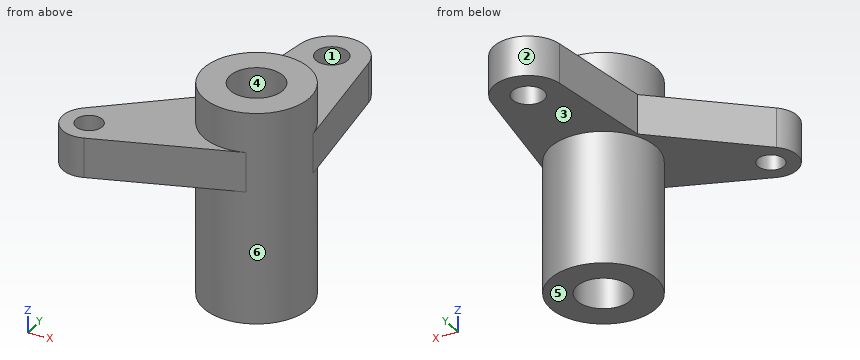
```python
from build123d import *

# Parameters (mm, degrees)
SKETCH_1_R      = 20
SKETCH_1_R_2    = 10
EXTRUDE_1_DEPTH = 80
EXTRUDE_START   = -15
SKETCH_1_3_R    = 13
SKETCH_1_3_R_2  = 6
SKETCH_1_3_R_3  = 10
SKETCH_1_3_R_4  = 5
EXTRUDE_2_DEPTH = 15


with BuildPart() as part:
    # Sketch 1 → Extrude 1 (new body)
    with BuildSketch(Plane.XY):
        Circle(SKETCH_1_R)
        Circle(SKETCH_1_R_2, mode=Mode.SUBTRACT)
    extrude(amount=-EXTRUDE_1_DEPTH)

    # Sketch 1_3 → Extrude 2 (add)
    # profile 1 of 5: a face of its own
    with BuildSketch(Plane.XY.offset(EXTRUDE_START)):
        with BuildLine():
            Line((-12.871969546, 51.82), (-18.742862332, 10.29804772))
            Line((-18.742862332, 10.29804772), (-12.982504947, 15.213630905))
            ThreePointArc((-12.982504947, 15.213630905), (7.081980571, 18.704158661), (19.803030071, 2.8))
            Line((19.803030071, 2.8), (12.871969546, 51.82))
            ThreePointArc((12.871969546, 51.82), (12.967952886, 50.912248842), (13, 50))
            ThreePointArc((13, 50), (-0.912248842, 37.032047114), (-12.871969546, 51.82))
        make_face()
    # profile 2 of 5: a face of its own
    with BuildSketch(Plane.XY.offset(EXTRUDE_START)):
        with BuildLine():
            Line((-12.982504947, 15.213630905), (-18.742862332, 10.29804772))
            Line((-18.742862332, 10.29804772), (-19.803030071, 2.8))
            ThreePointArc((-19.803030071, 2.8), (-17.528473541, 9.630815923), (-12.982504947, 15.213630905))
        make_face()
    # profile 3 of 5: a face of its own
    with BuildSketch(Plane.XY.offset(EXTRUDE_START)):
        with Locations((0, 50)):
            Circle(SKETCH_1_3_R)
        with Locations((0, 50)):
            Circle(SKETCH_1_3_R_2, mode=Mode.SUBTRACT)
    # profile 4 of 5: a face of its own
    with BuildSketch(Plane.XY.offset(EXTRUDE_START)):
        with BuildLine():
            Line((-18.742862332, 10.29804772), (-54.122649682, -19.893184548))
            ThreePointArc((-54.122649682, -19.893184548), (-43.442872691, -18.419456934), (-37.631397208, -27.5))
            ThreePointArc((-37.631397208, -27.5), (-39.463757039, -33.269718716), (-44.289328021, -36.924997271))
            Line((-44.289328021, -36.924997271), (6.684138374, -18.849994541))
            ThreePointArc((6.684138374, -18.849994541), (-12.657286271, -15.485254414), (-19.803030071, 2.8))
            Line((-19.803030071, 2.8), (-18.742862332, 10.29804772))
        make_face()
    # profile 5 of 5: a face of its own
    with BuildSketch(Plane.XY.offset(EXTRUDE_START)):
        with Locations((-47.631397208, -27.5)):
            Circle(SKETCH_1_3_R_3)
        with Locations((-47.631397208, -27.5)):
            Circle(SKETCH_1_3_R_4, mode=Mode.SUBTRACT)
    extrude(amount=-EXTRUDE_2_DEPTH)


solid = part.part
```
Could you check a few things on this model? Use its own coordinates, in mm. Face numbers are marked on the shaded views. A direction names the side the tool comes from. Coordinates: 2 decimals unless noted, no trailing zeros. Write each loop counter-clockwise with the first axis right and the second up, starting at its lowest first coordinate (ties: lowest second). Pieces come first, ordered by that corner, then holes. Notation, with made-up numbers: (50, 62.25) -> (101, 62.25) arc R37 ccw to (101, 101.25) -> close; hole circle Ø11 at (16, 32). An arc over 180 degrees is marked (long way). One line per question, with ' | ' between items. Start each with the question number.
1. If we section it at A-A (z = -25): Please give me the cut outline in (x, y) (3 decimals), and give its area (3 significant figures).
2. Thinking about a two-plate mould opening in Y: for the marked faces 1, 2, 3 and 4, which applies, pulls with the +Y half, pulls with the -Y half, needs draft (parallel to the pull), parting line crosses it, or undercut?
3. Please list where these lines run through material, in increasing order: line 1 along Y through (x, z) = (0, -42); line 2 along X through (y, z) = (-1, -42); line 3 along X through (y, z) = (47.5, -19).
4. Will these pins go through, and if not, where does the flat tip stop? P1, Ø10, axis at x = -20.5, y = 17, coming from the -Z side; P2, Ø4, axis at x = -8.5, z = -10.5, coming from the +Y side; P3, Ø12, axis at y = -13, z = -13, coming from the -X side.
5. For the marked faces 5 and 6, which set-ups out of +Z, -Z, +X, -X, +Y, -Y let a thin tool reach every point of the face, with its end or its side?
6. If we section it at B-B (y = 50): Please give me the cut outline in (x, z), and give its area (3 significant figures).
7. If we section it at D-D (x = 0): Please give me the cut outline in (y, z), and give its area (3 significant figures).
8. If we section it at C-C (z = -6): Please give me the cut outline in (x, y), and give its area (3 significant figures).
Return value:
1) outline: (-54.123, -19.893) arc R10 ccw to (-44.289, -36.925) -> (6.684, -18.85) arc R20 ccw to (19.803, 2.8) -> (12.872, 51.82) arc R13 ccw to (-12.872, 51.82) -> (-18.743, 10.298) -> close; hole circle Ø10 at (-47.631, -27.5); hole circle Ø20 at (0, 0); hole circle Ø12 at (0, 50) | area: 3,250 mm²
2) face 1: undercut | face 2: pulls with the +Y half | face 3: needs draft | face 4: undercut
3) line 1: y = -20 to -10, 10 to 20 | line 2: x = -19.97 to -9.95, 9.95 to 19.97 | line 3: x = -13.48 to -5.45, 5.45 to 13.48
4) P1: stops at z = -30 | P2: stops at y = 18.91 | P3: stops at x = -52.67
5) face 5: -Z, +X, -X, +Y, -Y | face 6: none
6) outline: (-13.13, -30) -> (-6, -30) -> (-6, -15) -> (-13.13, -15) -> close; (6, -30) -> (13.13, -30) -> (13.13, -15) -> (6, -15) -> close | area: 214 mm²
7) outline: (-21.22, -30) -> (-20, -30) -> (-20, -80) -> (-10, -80) -> (-10, 0) -> (-20, 0) -> (-20, -15) -> (-21.22, -15) -> close; (10, -80) -> (20, -80) -> (20, -30) -> (44, -30) -> (44, -15) -> (20, -15) -> (20, 0) -> (10, 0) -> close; (56, -30) -> (63, -30) -> (63, -15) -> (56, -15) -> close | area: 2,080 mm²
8) outline: circle Ø40 at (0, 0); hole circle Ø20 at (0, 0) | area: 942 mm²
